from build123d import *

# Parameters (mm, degrees)
ESQUISSE1_W             = 37
ESQUISSE1_H             = 20
ESQUISSE1_R             = 2.05
ESQUISSE1_R_2           = 1.6
BOSS_EXTRU_1_DEPTH      = 2.5
ESQUISSE3_R             = 1.6
ENL_V_MAT_EXTRU_1_DEPTH = 1
ENL_V_MAT_EXTRU_2_DEPTH = 1


with BuildPart() as part:
    # Esquisse1 → Boss.-Extru.1 (new body)
    with BuildSketch(Plane.XY):
        Rectangle(ESQUISSE1_W, ESQUISSE1_H)
        with Locations((-12, 6)):
            Circle(ESQUISSE1_R, mode=Mode.SUBTRACT)
        with Locations((-12, -6)):
            Circle(ESQUISSE1_R, mode=Mode.SUBTRACT)
        with Locations((15.5, 0)):
            Circle(ESQUISSE1_R, mode=Mode.SUBTRACT)
        with Locations((3.4, -1.5)):
            Circle(ESQUISSE1_R_2, mode=Mode.SUBTRACT)
        with BuildLine():
            Line((-3.738369819, -2.440040602), (0.723111318, -1.852515226))
            ThreePointArc((0.723111318, -1.852515226), (5.429936055, 0.280269534), (2.701188578, -4.107999731))
            Line((2.701188578, -4.107999731), (1.536502875, -8.454665949))
            ThreePointArc((1.536502875, -8.454665949), (8.813162812, 3.247385424), (-3.738369819, -2.440040602))
        make_face(mode=Mode.SUBTRACT)
    extrude(amount=BOSS_EXTRU_1_DEPTH)

    # Esquisse3 → Enlèv. mat.-Extru.1 (cut)
    # profile 1 of 2: a face of its own
    with BuildSketch(Plane(origin=(0, 0, 0), x_dir=(-1, 0, 0), z_dir=(0, 0, -1))):
        with BuildLine():
            Line((3.738369819, -2.440040602), (-0.723111318, -1.852515226))
            ThreePointArc((-0.723111318, -1.852515226), (-5.429936055, 0.280269534), (-2.701188578, -4.107999731))
            Line((-2.701188578, -4.107999731), (-1.536502875, -8.454665949))
            ThreePointArc((-1.536502875, -8.454665949), (-8.813162812, 3.247385424), (3.738369819, -2.440040602))
        make_face()
    # profile 2 of 2: a face of its own
    with BuildSketch(Plane(origin=(0, 0, 0), x_dir=(-1, 0, 0), z_dir=(0, 0, -1))):
        with BuildLine():
            Line((-2.118845727, -6.28133284), (1.50762925, -2.146277914))
            Line((1.50762925, -2.146277914), (-0.723111318, -1.852515226))
            ThreePointArc((-0.723111318, -1.852515226), (-5.429936055, 0.280269534), (-2.701188578, -4.107999731))
            Line((-2.701188578, -4.107999731), (-2.118845727, -6.28133284))
        make_face()
        with Locations((-3.4, -1.5)):
            Circle(ESQUISSE3_R, mode=Mode.SUBTRACT)
    extrude(amount=-ENL_V_MAT_EXTRU_1_DEPTH, mode=Mode.SUBTRACT)

    # Esquisse4 → Enlèv. mat.-Extru.2 (cut)
    with BuildSketch(Plane.XY.offset(2.5)):
        Polygon((-5.098492824, 2.565126725), (-3.402396632, 3.624965253), (-1.282719575, 0.232772869), (-2.978815767, -0.82706566), align=None)
        Polygon((11.151538443, 2.109938013), (12.565752005, 0.69572445), (9.73732488, -2.132702674), (8.323111318, -0.718489112), align=None)
        Polygon((10.086814623, -6.675295623), (9.569176533, -8.607147276), (5.705473228, -7.571871096), (6.223111318, -5.640019443), align=None)
    extrude(amount=-ENL_V_MAT_EXTRU_2_DEPTH, mode=Mode.SUBTRACT)


solid = part.part
Here's how the part is built. I have some questions about the finished solid (model axes, mm). A direction names the side the tool comes from. Round coordinates to 2 decimals unless told otherwise and drop trailing zeros. Loops run counter-clockwise (first coordinate to the right, second up) from the corner with the lowest first, then second, coordinate; pieces in that order, holes last. Notation, with made-up numbers: M 61,-11.75 L 90,-11.75 A21 ccw 90,10.25 Z; hole C 56.25,-16.5 d2. An arc over 180 degrees is marked long. Write each question's results on one line, items separated by ' | '. Start each with the question number.
(1) I want a section at A-A (x = 3.4). Please give me the cut outline in (y, z), then the cut area to 3 significant figures.
(2) Thinking about a two-plate mould opening in X: for faces 1 (the flat face through (0, -10, 1)), 2 (the flat face through (8.193, -8.238, 2.007)), 3 (the flat face through (18.5, 0, 1)), which applies, pulls with the +X half, pulls with the -X half, needs draft (parallel to the pull), parting line crosses it, or undercut?
(3) Will this pin go through, and if not, where does the flat tip stop? P1, Ø1.8, axis at x = 8.5, y = -7.5, coming from the +Z side.
(4) If I drill on probe 1 along Y at (x, z) = (3.4, 1.5); probe 2 along X at (y, z) = (-1.5, 0.35); probe 3 along Y at (x, z) = (3.4, 0.65), over which ranges is the centre line in solid material (lowest first)? Write a range as from..to.
(5) I want a section at C-C (z = 0.35). Please give me the cut outline in (x, y), then the cut area to 3 significant figures.
(6) I want a section at B-B (x = 15.5). Please give me the cut outline in (y, z).
(7) On a 3-axis mill with a long thin cutter (end or side, diameter ignored), from which of +Z, -Z, +X, -X, +Y, -Y can I reach the whole of each face in a straight line? I mean faces 4 (the flat face through (-2.035, -2.216, 1.51)), 5 (the flat face through (-4, 2, 1.5)), 6 (the flat face through (1.5, -2.5, 1)). Say none if no direction works.
(8) I want a section at D-D (x = -12). Please give me the cut outline in (y, z), then the cut area to 3 significant figures.
Solved:
1) outline: M -10,0 L -8.7,0 L -8.7,2.5 L -10,2.5 Z; M -4.2,1 L -3.1,1 L -3.1,2.5 L -4.2,2.5 Z; M 0.1,1 L 1.2,1 L 1.2,2.5 L 0.1,2.5 Z; M 5.7,0 L 10,0 L 10,2.5 L 5.7,2.5 Z | area: 17.3 mm²
2) face 1: needs draft | face 2: undercut | face 3: pulls with the +X half
3) P1: stops at z = 2.5
4) probe 1: y = -10..-8.7, -4.2..-3.1, 0.1..1.2, 5.7..10 | probe 2: x = -18.5..-3.8, 10.6..14.1, 16.9..18.5 | probe 3: y = -10..-8.7, 5.7..10
5) outline: M -18.5,-10 L 18.5,-10 L 18.5,10 L -18.5,10 Z; hole C -12,-6 d4.1; hole C -12,6 d4.1; hole M -3.74,-2.44 L -1.51,-2.15 L 2.12,-6.28 L 1.54,-8.45 A7.2 ccw long Z; hole C 15.5,0 d4.1 | area: 557 mm²
6) outline: M -10,0 L -2.05,0 L -2.05,2.5 L -10,2.5 Z; M 2.05,0 L 10,0 L 10,2.5 L 2.05,2.5 Z
7) face 4: +Z, -Z | face 5: +Z | face 6: -Z
8) outline: M -10,0 L -8.05,0 L -8.05,2.5 L -10,2.5 Z; M -3.95,0 L 3.95,0 L 3.95,2.5 L -3.95,2.5 Z; M 8.05,0 L 10,0 L 10,2.5 L 8.05,2.5 Z | area: 29.5 mm²
